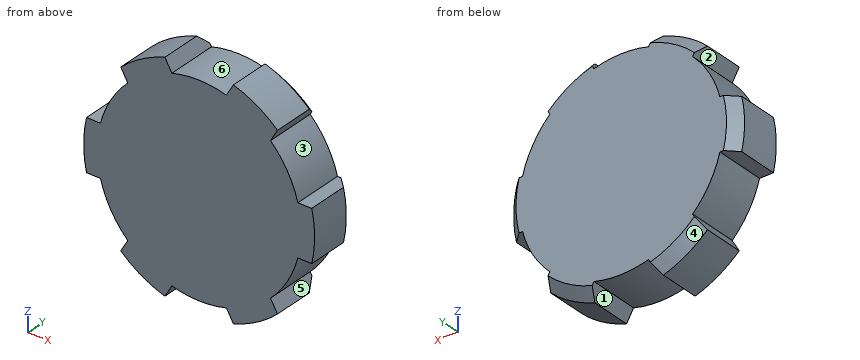
from build123d import *

# Parameters (mm, degrees)
SKETCH_1_R               = 10
EXTRUDE_1_DEPTH          = 5
EXTRUDE_2_DEPTH          = 5
PATTERN_CIRCULAR_1_COUNT = 3
PATTERN_CIRCULAR_1_ANGLE = 120
CHAMFER_1_SIZE           = 1


with BuildPart() as part:
    # 草图1 → 凸台-拉伸1 (new body)
    with BuildSketch(Plane(origin=(0, 0, 0), x_dir=(1, 0, 0), z_dir=(0, 1, 0))):
        Circle(SKETCH_1_R)
    extrude(amount=EXTRUDE_1_DEPTH)

    # 草图2 → 凸台-拉伸2 (add)
    with BuildSketch(Plane(origin=(0, 5, 0), x_dir=(1, 0, 0), z_dir=(0, 1, 0))):
        with BuildLine():
            Line((9.682458366, 2.5), (11.052828845, 2.5))
            ThreePointArc((11.052828845, 2.5), (11.332035363, 0), (11.052828845, -2.5))
            Line((11.052828845, -2.5), (9.682458366, -2.5))
            ThreePointArc((9.682458366, -2.5), (10, 0), (9.682458366, 2.5))
        make_face()
        with BuildLine():
            Line((-11.052828845, -2.5), (-9.682458366, -2.5))
            ThreePointArc((-9.682458366, -2.5), (-10, 0), (-9.682458366, 2.5))
            Line((-9.682458366, 2.5), (-11.052828845, 2.5))
            ThreePointArc((-11.052828845, 2.5), (-11.332035363, 0), (-11.052828845, -2.5))
        make_face()
    extrude_2 = extrude(amount=-EXTRUDE_2_DEPTH)

    # 阵列(圆周)1: 凸台-拉伸2 ×3 about axis
    pattern_circular_1_axis = Axis((0, 0, 0), (0, -1, 0))
    for i in range(1, PATTERN_CIRCULAR_1_COUNT):
        add(extrude_2.rotate(pattern_circular_1_axis, i * PATTERN_CIRCULAR_1_ANGLE / (PATTERN_CIRCULAR_1_COUNT - 1)))

    # 倒角1
    chamfer_1_edges = [part.edges().sort_by_distance(p)[0] for p in [
        (-11.332035363, 5, 0),
        (5.666017682, 5, 9.813830501),
        (-5.666017682, 5, -9.813830501),
        (-5.666017682, 5, 9.813830501),
        (5.666017682, 5, -9.813830501),
        (11.332035363, 5, 0),
    ]]
    chamfer(chamfer_1_edges, length=CHAMFER_1_SIZE)


solid = part.part
Verification items for the finished model (mm, model axes). Face numbers are marked on the shaded views. A direction names the side the tool comes from. Round coordinates to 2 decimals unless told otherwise and drop trailing zeros. Loops run counter-clockwise (first coordinate to the right, second up) from the corner with the lowest first, then second, coordinate; pieces in that order, holes last. Notation, with made-up numbers: (60.5, 27) - (111.5, 27) arc R13 cw to (111.5, 46) - close; hole circle Ø9 at (73, -28.5). An arc over 180 degrees is marked (long way). Use a Markdown table: item, result. Add a question column.
1. Section check D-D, the plane x = 8.75. Record the boundary of the cut face in (y, z).
2. Release check for a two-part mould opening along Z. For the marked faces 4, 5 and 6 record: released by +Z, released by -Z, zero draft, split by the parting line, or undercut.
3. Access from +Z, -Z, +X, -X, +Y, -Y to the whole of each face (thin tool, end or side, straight path). Record for the marked faces 1, 2 and 3.
4. Section check B-B, the plane z = -5.25. Record the boundary of the cut face in (x, y), plus the area to 3 significant figures.
5. Section check A-A, the plane y = 3.1. Record the boundary of the cut face in (x, z).
6. Thickness scan on probe 1 along X at (y, z) = (0.8, -7); probe 2 along X at (y, z) = (3.95, 0); probe 3 along Z at (x, y) = (0.25, 1.35). Record the ranges inside material, lowest first. Write a range as [from, to].
7. Gauge pin test, flat ends, axial feed: pin 1 (1.5 mm diameter, centred on x = -10, y = 3, fed in from +Z); pin 2 (1.5 mm diameter, centred on x = 10, y = 1.5, fed in from -Z); pin 3 (2 mm diameter, centred on x = -6, y = 2.5, fed in from +Z). Record the tip position at first contact, or that the pin passes through.
8. Section check C-C, the plane y = 4.3. Record the boundary of the cut face in (x, z), plus the area to 3 significant figures.
Checks:
| question | item | result |
|---|---|---|
| 1 | outline | (0, -4.84) - (5, -4.84) - (5, 4.84) - (0, 4.84) - close |
| 2 | face 4 | released by -Z |
| 2 | face 5 | undercut |
| 2 | face 6 | released by +Z |
| 3 | face 1 | -Z, +Y, -Y |
| 3 | face 2 | -X, +Y, -Y |
| 3 | face 3 | +X, +Y, -Y |
| 4 | outline | (-8.51, 0) - (8.51, 0) - (8.51, 5) - (-8.51, 5) - close |
| 4 | area | 85.1 mm^2 |
| 5 | outline | (-11.05, -2.5) - (-9.68, -2.5) arc R10 ccw to (-7.01, -7.14) - (-7.69, -8.32) arc R11.33 ccw to (-3.36, -10.82) - (-2.68, -9.64) arc R10 ccw to (2.68, -9.64) - (3.36, -10.82) arc R11.33 ccw to (7.69, -8.32) - (7.01, -7.14) arc R10 ccw to (9.68, -2.5) - (11.05, -2.5) arc R11.33 ccw to (11.05, 2.5) - (9.68, 2.5) arc R10 ccw to (7.01, 7.14) - (7.69, 8.32) arc R11.33 ccw to (3.36, 10.82) - (2.68, 9.64) arc R10 ccw to (-2.68, 9.64) - (-3.36, 10.82) arc R11.33 ccw to (-7.69, 8.32) - (-7.01, 7.14) arc R10 ccw to (-9.68, 2.5) - (-11.05, 2.5) arc R11.33 ccw to start |
| 6 | probe 1 | x = [-7.14, 7.14] |
| 6 | probe 2 | x = [-11.33, 11.33] |
| 6 | probe 3 | z = [-10, 10] |
| 7 | pin 1 | stops at z = 3.8 |
| 7 | pin 2 | stops at z = -3.8 |
| 7 | pin 3 | stops at z = 10.17 |
| 8 | outline | (-10.75, -2.5) - (-9.68, -2.5) arc R10 ccw to (-7.01, -7.14) - (-7.54, -8.06) arc R11.03 ccw to (-3.21, -10.56) - (-2.68, -9.64) arc R10 ccw to (2.68, -9.64) - (3.21, -10.56) arc R11.03 ccw to (7.54, -8.06) - (7.01, -7.14) arc R10 ccw to (9.68, -2.5) - (10.75, -2.5) arc R11.03 ccw to (10.75, 2.5) - (9.68, 2.5) arc R10 ccw to (7.01, 7.14) - (7.54, 8.06) arc R11.03 ccw to (3.21, 10.56) - (2.68, 9.64) arc R10 ccw to (-2.68, 9.64) - (-3.21, 10.56) arc R11.03 ccw to (-7.54, 8.06) - (-7.01, 7.14) arc R10 ccw to (-9.68, 2.5) - (-10.75, 2.5) arc R11.03 ccw to start |
| 8 | area | 345 mm^2 |
